CAD build for the part. Positions are in the model's coordinates, mm. Face numbers are marked on the shaded views. A direction names the side the tool comes from. Give positions to 0.01 mm unless a question says otherwise; leave off trailing zeros. Use one line per item in the form item = value. Start each with the question number.
from build123d import *

# Parameters (mm, degrees)
F0_W        = 83.5
F0_H        = 16.8
F1_DEPTH    = 9.5
F2_R        = 1.25
F3_DEPTH    = 25
F4_R        = 2.6
F4_R_2      = 1.05
F5_DEPTH    = 13.6
F6_R        = 1
F7_R        = 8
F8_SIZE2    = 1
F8_SIZE     = 3
F9_T1_DEPTH = 35.4784813046
F9_T3_DEPTH = 40.55


# Not quite as in the source:
# - a fillet or chamfer that OpenCascade refuses, or shapes differently, is made with other operations: its cross-section is extruded or revolved along the edge and cut away or added
# - a feature names something its author has since deleted; it is built from what else it names


with BuildPart() as f1:
    # F0 (on Front) → F1 (new body)
    with BuildSketch(Plane.XZ):
        Rectangle(F0_W, F0_H)
    extrude(amount=F1_DEPTH)

    # F2 (on face) → F3 (cut)
    with BuildSketch(Plane(origin=(0, 0, -8.4), x_dir=(1, 0, 0), z_dir=(0, 0, -1))):
        with Locations((-38.2, 5.95)):
            Circle(F2_R)
        Polygon((-18.75, 0), (-18.75, 4), (-41.75, 2.5), (-41.75, 0), align=None)
        with BuildLine():
            add(Edge.make_bspline(
                [(-18.75, 0), (-9.2352803439, 2.081155549), (4.6071284628, 1.7784279246), (15.029287035, 2.3336862795), (23.25, 1.4)],
                knots=[0, 0, 0, 0, 0.5257635341, 1, 1, 1, 1], degree=3))
            Line((-18.75, 0), (41.75, 0))
            Line((41.75, 0), (41.75, 2))
            Line((41.75, 2), (23.25, 1.4))
        make_face()
    extrude(amount=-F3_DEPTH, mode=Mode.SUBTRACT)

    # F4 (on face) → F5 (join)
    with BuildSketch(Plane(origin=(-0.0209275853, -0.6452672134, 0), x_dir=(-0.9994744832, 0.0324153886, 0), z_dir=(0.0324153886, 0.9994744832, 0))):
        with Locations((-31.7928904511, 0)):
            Circle(F4_R)
        with Locations((-31.7928904511, 0)):
            Circle(F4_R_2, mode=Mode.SUBTRACT)
    extrude(amount=F5_DEPTH)

    # F6
    f6_edges = [f1.edges().sort_by_distance(p)[0] for p in [
        (-18.75, -4, 0),
        (34.353889, -1.760126, 0),
        (-18.75, 0, 0),
    ]]
    fillet(f6_edges, radius=F6_R)

    # F7
    f7_edges = [f1.edges().sort_by_distance(p)[0] for p in [
        (41.75, -5.75, 8.4),
        (41.75, -5.75, -8.4),
    ]]
    fillet(f7_edges, radius=F7_R)

    # F8
    f8_edges = [f1.edges().sort_by_distance(p)[0] for p in [
        (-4, -9.5, 8.4),
    ]]
    f8_side = f1.faces().sort_by_distance((-0.798169, -9.5, 0))[0]
    chamfer(f8_edges, length=F8_SIZE, length2=F8_SIZE2, reference=f8_side)

    # F9: fillet of radius 3.5 on 2 edges, made by hand

    # F9_s2 → F9_t1 (cut)
    with BuildSketch(Plane.XY.offset(-17.7392406523)):
        with BuildLine():
            ThreePointArc((-41.75, -6.2356962609), (-40.6429877316, -3.6815604548), (-38.0222230193, -2.74311589))
            Line((-38.0222230193, -2.74311589), (-41.75, -2.5))
            Line((-41.75, -2.5), (-41.75, -6.2356962609))
        make_face()
    extrude(amount=F9_T1_DEPTH, mode=Mode.SUBTRACT)

    # F9_s4 → F9_t3 (cut)
    with BuildSketch(Plane.XY.offset(-20.275)):
        with BuildLine():
            ThreePointArc((-41.75, -6), (-40.7248737342, -8.4748737342), (-38.25, -9.5))
            Line((-38.25, -9.5), (-41.75, -9.5))
            Line((-41.75, -9.5), (-41.75, -6))
        make_face()
    extrude(amount=F9_T3_DEPTH, mode=Mode.SUBTRACT)


solid = f1.part
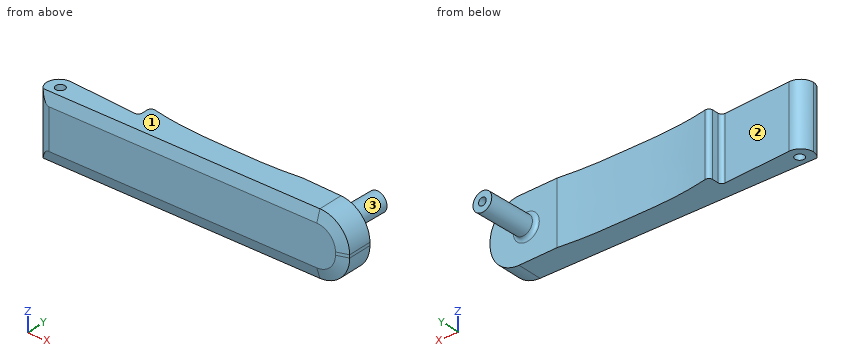
1) Pin check, flat tips, straight feed: pin 1 (5 mm diameter, centred on y = 7, z = -0.5, fed in from -X); pin 2 (0.8 mm diameter, centred on y = -2, z = 4, fed in from -X); pin 3 (4 mm diameter, centred on x = -23.5, z = 3.5, fed in from +Y); pin 4 (2 mm diameter, centred on x = -38.2, y = -5.95, fed in from -Z). Stop position of each tip, or through.
2) 3-axis set-ups, long thin cutter, end or side, ignore diameter. For the marked faces 1, 2 and 3: which of +Z, -Z, +X, -X, +Y, -Y reach the whole face in a straight line?
3) Wall check: line 1 along Y through (x, z) = (-38.2, 0.5); line 2 along Y through (x, z) = (23.5, 1.75); line 3 along X through (y, z) = (-5.95, -2.25). Give the ranges that are in metal, low to high. Write a range as from..to.
Final values:
q1.pin_1 = 29.36
q1.pin_2 = -18.75
q1.pin_3 = -3.56
q1.pin_4 = through
q2.face_1 = +Z, +X, -X, +Y, -Y
q2.face_2 = +Z, -Z, +Y
q2.face_3 = none
q3.line_1 = -9.5..-7.2, -4.7..-2.74
q3.line_2 = -9.5..-1.41
q3.line_3 = -41.74..-39.45, -36.95..41.53
